The model under review builds one solid part; all positions refer to its coordinate system, in mm. Round coordinates to 2 decimals unless told otherwise and drop trailing zeros. Loops run counter-clockwise (first coordinate to the right, second up) from the corner with the lowest first, then second, coordinate; pieces in that order, holes last. Notation, with made-up numbers: (34, -22) -> (49, -22) arc R32 cw to (49, 13) -> close; hole circle Ø7 at (-16.75, -13.5). An arc over 180 degrees is marked (long way). Use a Markdown table: item, result. Add a question column.
1) Wall thickness on probe 1 along Z at (x, y) = (-32, 40.25); probe 2 along Y at (x, z) = (-32.5, 5.5); probe 3 along X at (y, z) = (35.8, 6.35): over which ranges is each line inside the solid? List them lowest first.
2) Mouldability with a two-part tool opening along Z and no side actions: class faces 1 (the flat face through (-28, 41, 0)), 2 (the flat face through (-23.311, 36, 5)), 3 (the cylindrical face through (-28.801, 40.988, 2.603)) as released by +Z, released by -Z, zero draft, split by the parting line, or undercut.
3) Consider section C-C on y = 43.5. Give the boundary of the cut face in (x, z).
4) Insertion check: pin 1 (3 mm diameter, centred on x = -30, z = 7.5, fed in from +Y). The pin has a flat end and moves straight along its axis. Give the tip position at first contact, or say it passes through.
5) Consider section B-B on x = -27.25. Give the boundary of the cut face in (y, z).
6) Consider section A-A on z = 6.35. Give the boundary of the cut face in (x, y), plus the area to 3 significant figures.
7) Consider section D-D on y = 40.5. Give the boundary of the cut face in (x, z).
from build123d import *

# Parameters (mm, degrees)
F0_W     = 10.828417
F0_H     = 10.828416
F1_DEPTH = 12.7
F2_R     = 3.838495
F3_DEPTH = 25.4
F4_R     = 3.386017
F5_DEPTH = 25.4
F6_R     = 1.27


with BuildPart() as f1:
    # F0 (on Top) → F1 (new body)
    with BuildSketch(Plane.XY):
        with Locations((-28.725398, 40.155394)):
            Rectangle(F0_W, F0_H)
    extrude(amount=F1_DEPTH)

    # F2 (on face) → F3 (cut)
    with BuildSketch(Plane(origin=(-34.139607, 0, 0), x_dir=(0, -1, 0), z_dir=(-1, 0, 0))):
        with Locations((-40.155394, 6.35)):
            Circle(F2_R)
    extrude(amount=-F3_DEPTH, mode=Mode.SUBTRACT)

    # F4 (on face) → F5 (cut)
    with BuildSketch(Plane(origin=(0, 45.569602, 0), x_dir=(-1, 0, 0), z_dir=(0, 1, 0))):
        with Locations((28.725399, 6.35)):
            Circle(F4_R)
    extrude(amount=-F5_DEPTH, mode=Mode.SUBTRACT)

    # F6
    f6_edges = [f1.edges().sort_by_distance(p)[0] for p in [
        (-34.139607, 40.155394, 12.7),
        (-34.139607, 45.569602, 6.35),
        (-34.139607, 40.155394, 0),
        (-34.139607, 34.741186, 6.35),
        (-28.725399, 34.741186, 12.7),
        (-28.725399, 34.741186, 0),
    ]]
    fillet(f6_edges, radius=F6_R)


solid = f1.part
Result set:
| question | item | result |
|---|---|---|
| 1 | probe 1 | 0 to 2.51, 10.19 to 12.7 |
| 1 | probe 2 | 34.74 to 36.41, 43.9 to 45.57 |
| 1 | probe 3 | -34.12 to -32.11, -25.34 to -23.31 |
| 2 | face 1 | released by -Z |
| 2 | face 2 | zero draft |
| 2 | face 3 | undercut |
| 3 | outline | (-34.14, 1.27) arc R1.27 ccw to (-32.87, 0) -> (-23.31, 0) -> (-23.31, 4.47) -> (-25.91, 4.47) arc R3.39 cw to (-31.54, 4.47) -> (-34.14, 4.47) -> close; (-34.14, 8.23) -> (-31.54, 8.23) arc R3.39 cw to (-25.91, 8.23) -> (-23.31, 8.23) -> (-23.31, 12.7) -> (-32.87, 12.7) arc R1.27 ccw to (-34.14, 11.43) -> close |
| 4 | pin 1 | through |
| 5 | outline | (34.74, 1.27) arc R1.27 ccw to (36.01, 0) -> (45.57, 0) -> (45.57, 3.3) -> (42.49, 3.3) arc R3.84 cw to (37.82, 3.3) -> (34.74, 3.3) -> close; (34.74, 9.4) -> (37.82, 9.4) arc R3.84 cw to (42.49, 9.4) -> (45.57, 9.4) -> (45.57, 12.7) -> (36.01, 12.7) arc R1.27 ccw to (34.74, 11.43) -> close |
| 6 | outline | (-34.14, 36.01) arc R1.27 ccw to (-32.87, 34.74) -> (-32.11, 34.74) -> (-32.11, 36.32) -> (-34.14, 36.32) -> close; (-34.14, 43.99) -> (-32.11, 43.99) -> (-32.11, 45.57) -> (-32.87, 45.57) arc R1.27 ccw to (-34.14, 44.3) -> close; (-25.34, 34.74) -> (-23.31, 34.74) -> (-23.31, 36.32) -> (-25.34, 36.32) -> close; (-25.34, 43.99) -> (-23.31, 43.99) -> (-23.31, 45.57) -> (-25.34, 45.57) -> close |
| 6 | area | 12.1 mm2 |
| 7 | outline | (-34.14, 1.27) arc R1.27 ccw to (-32.87, 0) -> (-23.31, 0) -> (-23.31, 2.53) -> (-34.14, 2.53) -> close; (-34.14, 10.17) -> (-23.31, 10.17) -> (-23.31, 12.7) -> (-32.87, 12.7) arc R1.27 ccw to (-34.14, 11.43) -> close |
